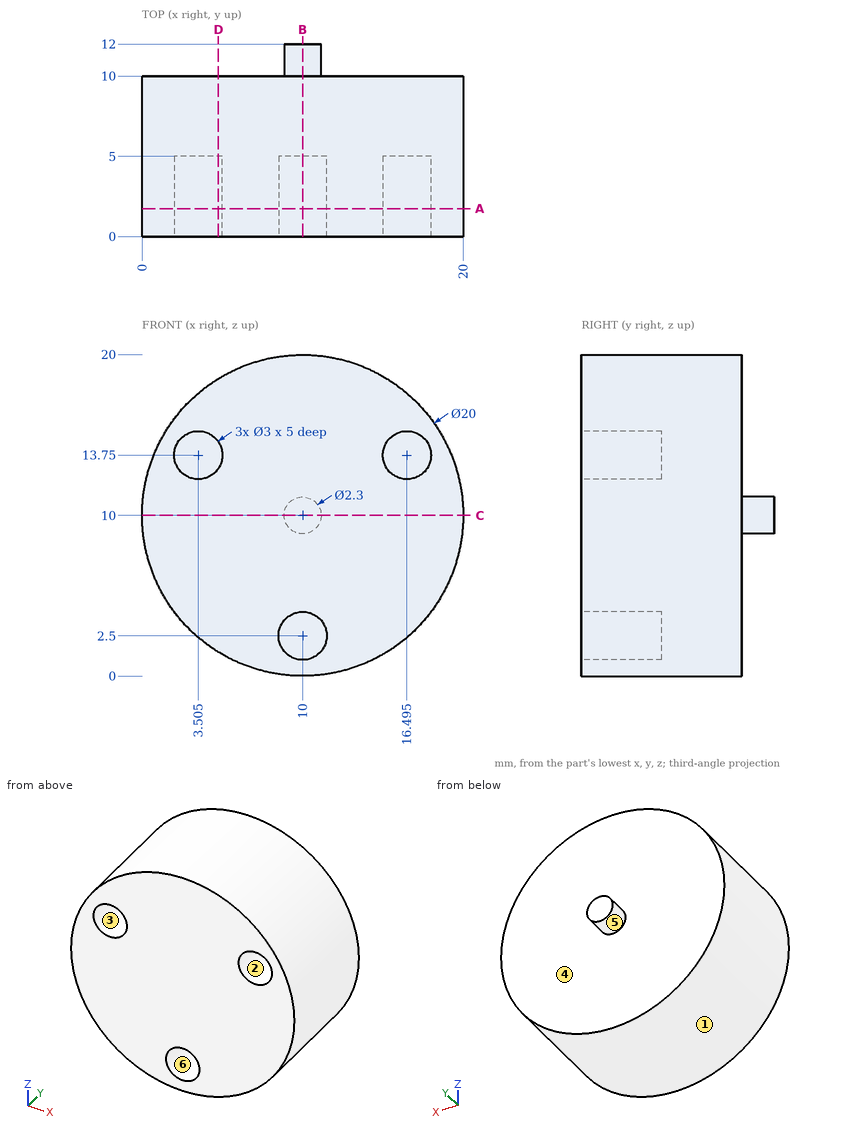
Design review of the part shown in the three views and the two pictorial views. Dimensions are in mm from the part's minimum x, y and z. A direction names the side the tool comes from. Give positions to 0.01 mm unless a question says otherwise; leave off trailing zeros. Loops run counter-clockwise (first coordinate to the right, second up) from the corner with the lowest first, then second, coordinate; pieces in that order, holes last. Notation, with made-up numbers: (45, -2) -> (74, -2) arc R13 ccw to (74, 5) -> close; hole circle Ø11 at (48, 70). An arc over 180 degrees is marked (long way). Answer as a JSON object with one key per item and string values. Group by question number.
Q1. Take a section at B-B (x = 10). Write out the cut boundary in (y, z), plus the area to 3 significant figures.
Q2. Take a section at D-D (x = 4.75). Write out the cut boundary in (y, z), plus the area to 3 significant figures.
Q3. Draft analysis for pull direction X (two halves, no side actions). For the marked faces 3, 4, 5 and 6, state which applies: pulls with the +X half, pulls with the -X half, needs draft (parallel to the pull), parting line crosses it, or undercut.
Q4. Tool access review of the marked faces 1 and 2: name each direction out of +Z, -Z, +X, -X, +Y, -Y from which nothing blocks a thin tool from reaching the whole face with its end or side.
Q5. Insertion check: pin 1 (3 mm diameter, centred on y = 4.5, z = 17.5, fed in from -X); pin 2 (5 mm diameter, centred on x = 5, z = 4.5, fed in from +Y); pin 3 (2 mm diameter, centred on y = 1.5, z = 3.5, fed in from +X). Each pin has a flat end and moves straight along its axis. Give the tip position at first contact, or say it passes through.
Q6. Take a section at C-C (z = 10). Write out the cut boundary in (x, y), plus the area to 3 significant figures.
Q7. Take a section at A-A (y = 1.75). State how many separate pieces and enclosed holes the cut face has, plus the area to 3 significant figures.
Q8. Wall thickness on line 1 along X through (y, z) = (1.4, 13.75) (1 decimal); line 2 along Z through (x, y) = (10, 2.6); line 3 along Y through (x, z) = (17.25, 13.75): over which ranges is each line inside the solid? List them lowest first.
Answer below:
{
 "1": {"outline": "(0, 0) -> (10, 0) -> (10, 8.85) -> (12, 8.85) -> (12, 11.15) -> (10, 11.15) -> (10, 20) -> (0, 20) -> (0, 4) -> (5, 4) -> (5, 1) -> (0, 1) -> close", "area": "190 mm2"},
 "2": {"outline": "(0, 1.49) -> (10, 1.49) -> (10, 18.51) -> (0, 18.51) -> (0, 14.59) -> (5, 14.59) -> (5, 12.91) -> (0, 12.91) -> close", "area": "162 mm2"},
 "3": {"face 3": "undercut", "face 4": "needs draft", "face 5": "parting line crosses it", "face 6": "undercut"},
 "4": {"face 1": "+Y, -Y", "face 2": "-Y"},
 "5": {"pin 1": "stops at x = 2", "pin 2": "stops at y = 10", "pin 3": "stops at x = 18.35"},
 "6": {"outline": "(0, 0) -> (20, 0) -> (20, 10) -> (11.15, 10) -> (11.15, 12) -> (8.85, 12) -> (8.85, 10) -> (0, 10) -> close", "area": "205 mm2"},
 "7": {"separate pieces": "1", "enclosed holes": "3", "area": "293 mm2"},
 "8": {"line 1": "x = 0.7 to 2, 5 to 15, 18 to 19.3", "line 2": "z = 0 to 1, 4 to 20", "line 3": "y = 5 to 10"}
}
